```python
from build123d import *

# Parameters (mm, degrees)
SKETCH1_W           = 149
SKETCH1_H           = 65
BOSS_EXTRUDE1_DEPTH = 3
SKETCH2_W           = 149
SKETCH2_H           = 65
SKETCH2_W_2         = 143
SKETCH2_H_2         = 59
BOSS_EXTRUDE2_DEPTH = 50
BOSS_EXTRUDE3_DEPTH = 50
SKETCH5_R           = 2
CUT_EXTRUDE1_DEPTH  = 3


with BuildPart() as part:
    # Sketch1 → Boss-Extrude1 (new body)
    with BuildSketch(Plane.XY):
        with Locations((74.5, -32.5)):
            Rectangle(SKETCH1_W, SKETCH1_H)
    extrude(amount=BOSS_EXTRUDE1_DEPTH)

    # Sketch2 → Boss-Extrude2 (add)
    with BuildSketch(Plane.XY.offset(3)):
        with Locations((74.5, -32.5)):
            Rectangle(SKETCH2_W, SKETCH2_H)
        with Locations((74.5, -32.5)):
            Rectangle(SKETCH2_W_2, SKETCH2_H_2, mode=Mode.SUBTRACT)
    extrude(amount=BOSS_EXTRUDE2_DEPTH)

    # Sketch4 → Boss-Extrude3 (add)
    with BuildSketch(Plane.XY.offset(3)):
        Polygon((73, -3), (73, -31), (3, -31), (3, -34), (73, -34), (73, -62), (76, -62), (76, -34), (146, -34), (146, -31), (76, -31), (76, -3), align=None)
    extrude(amount=BOSS_EXTRUDE3_DEPTH)

    # Sketch5 → Cut-Extrude1 (cut)
    with BuildSketch(Plane(origin=(0, 0, 0), x_dir=(1, 0, 0), z_dir=(0, 1, 0))):
        with Locations(Location((39.5, -28, 0), (0, 0, 270))):
            Circle(SKETCH5_R)
        with Locations(Location((109.5, -28, 0), (0, 0, 270))):
            Circle(SKETCH5_R)
    extrude(amount=-CUT_EXTRUDE1_DEPTH, mode=Mode.SUBTRACT)


solid = part.part
```
Design review of the part built by this model. Coordinates are the model's own, in mm. A direction names the side the tool comes from. Round coordinates to 2 decimals unless told otherwise and drop trailing zeros. Order: outer loops, then holes, each group sorted by start corner. A loop starts at its lowest first (then second) coordinate and runs counter-clockwise, first axis right, second up. Notation, with made-up numbers: (52, 49) - (92, 49) arc R25 ccw to (92, 88) - close; hole circle Ø6 at (-39.5, 19.25). An arc over 180 degrees is marked (long way). One line per question, with ' | ' between items.
Item 1: Take a section at C-C, the plane z = 28. Write out the cut boundary in (x, y), then the cut area to 3 significant figures.
Checks:
outline: (0, -65) - (149, -65) - (149, 0) - (111.5, 0) - (111.5, -3) - (146, -3) - (146, -31) - (76, -31) - (76, -3) - (107.5, -3) - (107.5, 0) - (41.5, 0) - (41.5, -3) - (73, -3) - (73, -31) - (3, -31) - (3, -3) - (37.5, -3) - (37.5, 0) - (0, 0) - close; hole (3, -62) - (73, -62) - (73, -34) - (3, -34) - close; hole (76, -62) - (146, -62) - (146, -34) - (76, -34) - close | area: 1,820 mm²
Item 2: For P1, Ø1, axis at x = 108, y = -16.5, coming from the +Z side, flat-tipped, find the tip position at first contact; note if it passes through.
Checks:
P1: z = 3
Item 3: Take a section at D-D, the plane y = -41.5. Write out the cut boundary in (x, z).
Checks:
outline: (0, 0) - (149, 0) - (149, 53) - (146, 53) - (146, 3) - (76, 3) - (76, 53) - (73, 53) - (73, 3) - (3, 3) - (3, 53) - (0, 53) - close
Item 4: Machinability: for faces 1 (the face through (37.726, -1.479, 28.923)), 2 (the face through (38, -17, 3)), 3 (the face through (149, -33, 26)), which of the approach directions +Z, -Z, +X, -X, +Y, -Y give a long, thin tool a straight path to every point of the face, cutting with its end or side? Answer none if there is none.
Checks:
face 1: +Y | face 2: +Z | face 3: +Z, -Z, +X, +Y, -Y
Item 5: Take a section at A-A, the plane x = 39.5. Write out the cut boundary in (y, z).
Checks:
outline: (-65, 0) - (0, 0) - (0, 26) - (-3, 26) - (-3, 3) - (-31, 3) - (-31, 53) - (-34, 53) - (-34, 3) - (-62, 3) - (-62, 53) - (-65, 53) - close; (-3, 30) - (0, 30) - (0, 53) - (-3, 53) - close
Item 6: Wall thickness on line 1 (Y direction, x = 48, z = 38); line 2 (X direction, y = -1, z = 28); line 3 (X direction, y = -20, z = 22.5): over which ranges is each line inside the solid? List them lowest first. Write a range as [from, to].
Checks:
line 1: [-65, -62], [-34, -31], [-3, 0] | line 2: [0, 37.5], [41.5, 107.5], [111.5, 149] | line 3: [0, 3], [73, 76], [146, 149]
Item 7: Draft analysis for pull direction Y (two halves, no side actions). For faces 4 (the face through (73, -65, 26)), 5 (the face through (111, -31, 28)), 6 (the face through (0, -33, 26)), state which applies: +Y half, -Y half, draft (parallel to the pull), parting line (faces both ways), or undercut.
Checks:
face 4: -Y half | face 5: undercut | face 6: draft
Item 8: Take a section at B-B, the plane z = 14.5. Write out the cut boundary in (x, y).
Checks:
outline: (0, -65) - (149, -65) - (149, 0) - (0, 0) - close; hole (3, -62) - (73, -62) - (73, -34) - (3, -34) - close; hole (3, -31) - (73, -31) - (73, -3) - (3, -3) - close; hole (76, -62) - (146, -62) - (146, -34) - (76, -34) - close; hole (76, -31) - (146, -31) - (146, -3) - (76, -3) - close
